Could you check a few things on this model? Use its own coordinates, in mm. A direction names the side the tool comes from. Round coordinates to 2 decimals unless told otherwise and drop trailing zeros. Write each loop counter-clockwise with the first axis right and the second up, starting at its lowest first coordinate (ties: lowest second). Pieces come first, ordered by that corner, then holes.
```python
from build123d import *

# Parameters (mm, degrees)
SKETCH1_W                                    = 60
SKETCH1_H                                    = 8
BOSS_EXTRUDE1_DEPTH                          = 120
CBORE_FOR_M3_HEX_SOCKET_HEAD_CAP_SCR_2_COUNT = 2
CBORE_FOR_M3_HEX_SOCKET_HEAD_CAP_SCR_2_PITCH = 40
CBORE_FOR_M3_HEX_SOCKET_HEAD_CAP_SCR_3_COUNT = 2
CBORE_FOR_M3_HEX_SOCKET_HEAD_CAP_SCR_3_PITCH = 60
CBORE_FOR_M3_HEX_SOCKET_HEAD_CAP_SCR_4_COUNT = 2
CBORE_FOR_M3_HEX_SOCKET_HEAD_CAP_SCR_4_PITCH = 80
CBORE_FOR_M3_HEX_SOCKET_HEAD_CAP_SCR_5_COUNT = 2
CBORE_FOR_M3_HEX_SOCKET_HEAD_CAP_SCR_5_PITCH = 20


with BuildPart() as part:
    # Sketch1 → Boss-Extrude1 (new body)
    with BuildSketch(Plane.XY):
        with Locations((30, 4)):
            Rectangle(SKETCH1_W, SKETCH1_H)
    extrude(amount=BOSS_EXTRUDE1_DEPTH)

    # Sketch4 → CBORE for M3 Hex Socket Head Cap Screw1 (revolve, cut)
    with BuildSketch(Plane(origin=(17.101413203, 0, 100), x_dir=(0, 0, -1), z_dir=(1, 0, 0))):
        Polygon((0, 0), (0, 7.021463052), (1.7, 6), (1.7, 3.4), (3.25, 3.4), (3.25, 0.025), (3.275, 0), align=None)
    cbore_for_m3_hex_socket_head_cap_screw1 = revolve(axis=Axis((17.101413203, -6.35, 100), (0, 1, 0)), mode=Mode.SUBTRACT)

    # CBORE for M3 Hex Socket Head Cap Scr 2: CBORE for M3 Hex Socket Head Cap Screw1 ×2
    with Locations(*[(0, 0, -i * CBORE_FOR_M3_HEX_SOCKET_HEAD_CAP_SCR_2_PITCH) for i in range(1, CBORE_FOR_M3_HEX_SOCKET_HEAD_CAP_SCR_2_COUNT)]):
        add(cbore_for_m3_hex_socket_head_cap_screw1, mode=Mode.SUBTRACT)

    # CBORE for M3 Hex Socket Head Cap Scr 3: CBORE for M3 Hex Socket Head Cap Screw1 ×2
    with Locations(*[(0, 0, -i * CBORE_FOR_M3_HEX_SOCKET_HEAD_CAP_SCR_3_PITCH) for i in range(1, CBORE_FOR_M3_HEX_SOCKET_HEAD_CAP_SCR_3_COUNT)]):
        add(cbore_for_m3_hex_socket_head_cap_screw1, mode=Mode.SUBTRACT)

    # CBORE for M3 Hex Socket Head Cap Scr 4: CBORE for M3 Hex Socket Head Cap Screw1 ×2
    with Locations(*[(0, 0, -i * CBORE_FOR_M3_HEX_SOCKET_HEAD_CAP_SCR_4_PITCH) for i in range(1, CBORE_FOR_M3_HEX_SOCKET_HEAD_CAP_SCR_4_COUNT)]):
        add(cbore_for_m3_hex_socket_head_cap_screw1, mode=Mode.SUBTRACT)

    # CBORE for M3 Hex Socket Head Cap Scr 5: CBORE for M3 Hex Socket Head Cap Screw1 ×2
    with Locations(*[(0, 0, -i * CBORE_FOR_M3_HEX_SOCKET_HEAD_CAP_SCR_5_PITCH) for i in range(1, CBORE_FOR_M3_HEX_SOCKET_HEAD_CAP_SCR_5_COUNT)]):
        add(cbore_for_m3_hex_socket_head_cap_screw1, mode=Mode.SUBTRACT)


solid = part.part
```
Q1. Imagine slicing it at A-A, the plane y = 1.75. Write out the boundary of the cut face in (x, z), then the cut area to 3 significant figures.
Q2. We'd pull the mould along Z, two halves only. Please class faces 1 (the flat face through (60, 4, 59)), 2 (the conical face through (17.214, 6.844, 39.727)): pulls with the +Z half, pulls with the -Z half, needs draft (parallel to the pull), parting line crosses it, or undercut.
Q3. If I drill on L1, parallel to Z at x = 17, y = 5.75; L2, parallel to Z at x = 18.5, y = 4.5; L3, parallel to X at y = 2.3, z = 40, over which ranges is the centre line in solid material (lowest first)?
Q4. I'm going to push flat-ended pins straight in: pin 1 Ø2.5 at (x, z) = (17.1, 80) entering from -Y; pin 2 Ø2 at (x, z) = (16, 99.5) entering from -Y; pin 3 Ø2 at (x, z) = (17, 20) entering from -Y. Where does each tip first touch, or does it pass through?
Q5. On a 3-axis mill with a long thin cutter (end or side, diameter ignored), from which of +Z, -Z, +X, -X, +Y, -Y can I reach the whole of each face in a straight line? I mean faces 3 (the cylindrical face through (16.59, 4.68, 18.38)), 4 (the flat face through (30, 0, 59)). Say none if no direction works.
Results found:
1. outline: (0, 0) - (60, 0) - (60, 120) - (0, 120) - close; hole circle Ø6.5 at (17.1, 20); hole circle Ø6.5 at (17.1, 40); hole circle Ø6.5 at (17.1, 60); hole circle Ø6.5 at (17.1, 80); hole circle Ø6.5 at (17.1, 100)
1. area: 7,030 mm2
2. face 1: needs draft
2. face 2: undercut
3. L1: z = 0 to 18.3, 21.7 to 38.3, 41.7 to 58.3, 61.7 to 78.3, 81.7 to 98.3, 101.7 to 120
3. L2: z = 0 to 19.03, 20.97 to 39.03, 40.97 to 59.03, 60.97 to 79.03, 80.97 to 99.03, 100.97 to 120
3. L3: x = 0 to 13.85, 20.35 to 60
4. pin 1: stops at y = 6.27
4. pin 2: stops at y = 3.4
4. pin 3: stops at y = 6.36
5. face 3: -Y
5. face 4: +Z, -Z, +X, -X, -Y
